Work out the finished part from the listing and answer in its coordinate system (mm). Face numbers are marked on the shaded views. A direction names the side the tool comes from. Coordinates: 2 decimals unless noted, no trailing zeros. Write each loop counter-clockwise with the first axis right and the second up, starting at its lowest first coordinate (ties: lowest second). Pieces come first, ordered by that corner, then holes. Notation, with made-up numbers: (55.5, 62.25) - (110.5, 62.25) arc R23 cw to (110.5, 79.25) - close; hole circle Ø7 at (44.25, -23). An arc over 180 degrees is marked (long way). One line per item, written item: value.
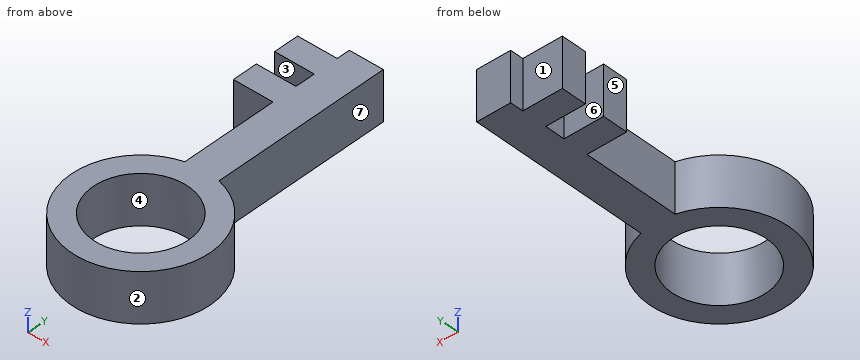
Autodesk Inventor part; units mm, degrees
ref_plane "YZ Plane" through (0, 0, 0) normal (1, 0, 0) x (0, 1, 0)
ref_plane "XZ Plane" through (0, 0, 0) normal (0, 1, 0) x (-1, 0, 0)
ref_plane "XY Plane" through (0, 0, 0) normal (0, 0, 1) x (1, 0, 0)
sketch "Sketch1" plane through (0, 0, 0) normal (0, 0, 1) x (1, 0, 0)
  arc A0 (-2.6945, 10.3961) -> (2.5563, 10.431) centre (0, 0) ccw
  circle A1 centre (0, 0) radius 7.3439
  line L0 (-2.6945, 38.1942) -> (2.5563, 38.1942)
  line L1 (-8.8208, 36.1476) -> (-2.6945, 36.1476)
  line L2 (-2.6945, 32.2644) -> (-8.8208, 32.2644)
  line L3 (-8.8208, 32.2644) -> (-8.8208, 36.1476)
  line L4 (-8.8208, 29.1799) -> (-2.6945, 29.1799)
  line L5 (-2.6945, 25.2966) -> (-8.8208, 25.2966)
  line L6 (-8.8208, 25.2966) -> (-8.8208, 29.1799)
  line L7 (-2.6945, 36.1476) -> (-2.6945, 38.1942)
  line L8 (-2.6945, 29.1799) -> (-2.6945, 32.2644)
  line L9 (-2.6945, 10.3961) -> (-2.6945, 25.2966)
  line L10 (2.5563, 38.1942) -> (2.5563, 10.431)
extrude "Extrusion1" add sketch "Sketch1" along normal blind 7.62
properties part number "Key"
Item 1: Section B-B, the plane x = 0 is taken. Determine the outline of the cut face in (y, z).
Evaluation:
outline: (-10.74, 0) - (-7.34, 0) - (-7.34, 7.62) - (-10.74, 7.62) - close; (7.34, 0) - (38.19, 0) - (38.19, 7.62) - (7.34, 7.62) - close
Item 2: Determine the mould class of the marked faces 4, 5, 6 and 7 for opening direction X: +X half, -X half, draft (parallel to the pull), parting line (faces both ways), or undercut.
Evaluation:
face 4: undercut
face 5: -X half
face 6: draft
face 7: +X half
Item 3: Section A-A, the plane z = 1.25 is taken. Determine the outline of the cut face in (x, y).
Evaluation:
outline: (-8.82, 25.3) - (-2.69, 25.3) - (-2.69, 10.4) arc R10.74 ccw (long way) to (2.56, 10.43) - (2.56, 38.19) - (-2.69, 38.19) - (-2.69, 36.15) - (-8.82, 36.15) - (-8.82, 32.26) - (-2.69, 32.26) - (-2.69, 29.18) - (-8.82, 29.18) - close; hole circle Ø14.69 at (0, 0)
Item 4: Which of the six approach directions +Z, -Z, +X, -X, +Y, -Y give full straight-line access (tool end or side, diameter ignored) to the marked faces 1, 2 and 3?
Evaluation:
face 1: +Z, -Z, -X, +Y
face 2: +Z, -Z
face 3: +Z, -Z, -X
Item 5: Section C-C, the plane y = 0 is taken. Determine the outline of the cut face in (x, z), then the cut area to 3 significant figures.
Evaluation:
outline: (-10.74, 0) - (-7.34, 0) - (-7.34, 7.62) - (-10.74, 7.62) - close; (7.34, 0) - (10.74, 0) - (10.74, 7.62) - (7.34, 7.62) - close
area: 51.8 mm2
Item 6: Consider probe 1 along Y at (x, z) = (0, 2); probe 2 along X at (y, z) = (17.5, 5.5); probe 3 along X at (y, z) = (-6.5, 3.5). Determine where each line is inside the solid, lowest interval first.
Evaluation:
probe 1: y = -10.74 to -7.34, 7.34 to 38.19
probe 2: x = -2.69 to 2.56
probe 3: x = -8.55 to -3.42, 3.42 to 8.55
Item 7: Given pin 1 (4 mm diameter, centred on y = 19.5, z = 5, fed in from -X); pin 2 (4 mm diameter, centred on y = 28.5, z = 4.5, fed in from -X); pin 3 (1.8 mm diameter, centred on x = -7.5, z = 5, fed in from +Y), each flat-ended and moving along its own axis, determine where each tip first touches the part or whether it passes through.
Evaluation:
pin 1: stops at x = -2.69
pin 2: stops at x = -8.82
pin 3: stops at y = 36.15
Item 8: Section D-D, the plane x = -3.5 is taken. Determine the outline of the cut face in (y, z), then the cut area to 3 significant figures.
Evaluation:
outline: (-10.15, 0) - (-6.46, 0) - (-6.46, 7.62) - (-10.15, 7.62) - close; (6.46, 0) - (10.15, 0) - (10.15, 7.62) - (6.46, 7.62) - close; (25.3, 0) - (29.18, 0) - (29.18, 7.62) - (25.3, 7.62) - close; (32.26, 0) - (36.15, 0) - (36.15, 7.62) - (32.26, 7.62) - close
area: 116 mm2
